from build123d import *

# Parameters (mm, degrees)
Y_KSEKLIK_EKSTR_ZYON1_DEPTH = 9
IZIM2_R                     = 1
KES_EKSTR_ZYON1_DEPTH       = 9
L_EK1_SCALE                 = 0.5


with BuildPart() as part:
    # Çizim1 → Yükseklik-Ekstrüzyon1 (new body)
    with BuildSketch(Plane(origin=(0, 0, 0), x_dir=(1, 0, 0), z_dir=(0, 1, 0))):
        with BuildLine():
            Line((3.94, 0), (3.94, -1.970806212))
            ThreePointArc((3.94, -1.970806212), (4.455977206, -3.302963323), (5.734671586, -3.94))
            Line((5.734671586, -3.94), (11.94, -3.94))
            Line((11.94, -3.94), (11.94, -1.970806212))
            Line((11.94, -1.970806212), (7.888485675, -1.970806212))
            ThreePointArc((7.888485675, -1.970806212), (6.494915238, -1.393570437), (5.917679463, 0))
            ThreePointArc((5.917679463, 0), (0, 5.917679463), (-5.917679463, 0))
            ThreePointArc((-5.917679463, 0), (-6.494915238, -1.393570437), (-7.888485675, -1.970806212))
            Line((-7.888485675, -1.970806212), (-11.94, -1.970806212))
            Line((-11.94, -1.970806212), (-11.94, -3.941612423))
            Line((-11.94, -3.941612423), (-5.752940471, -3.941612423))
            ThreePointArc((-5.752940471, -3.941612423), (-4.462169762, -3.309726511), (-3.94, -1.970806212))
            Line((-3.94, -1.970806212), (-3.94, 0))
            ThreePointArc((-3.94, 0), (0, 3.94), (3.94, 0))
        make_face()
    extrude(amount=Y_KSEKLIK_EKSTR_ZYON1_DEPTH)

    # Çizim2 → Kes-Ekstrüzyon1 (cut)
    with BuildSketch(Plane(origin=(0, 0, 1.970806212), x_dir=(-1, 0, 0), z_dir=(0, 0, -1))):
        with Locations((-9.914242837, 6.75)):
            Circle(IZIM2_R)
        with Locations((-9.914242837, 2.25)):
            Circle(IZIM2_R)
        with Locations((9.914242837, 2.25)):
            Circle(IZIM2_R)
        with Locations((9.914242837, 6.75)):
            Circle(IZIM2_R)
    extrude(amount=-KES_EKSTR_ZYON1_DEPTH, mode=Mode.SUBTRACT)


with BuildPart() as part_1:
    # Ölçek1: scaled about (-0.001148425, 4.5, -0.117296344)
    add(part.part.scale(L_EK1_SCALE).moved(Location((-0.000574213, 2.25, -0.058648172))))


solid = part_1.part
Read the model definition and answer for the solid it produces. Units are mm, in the model's axes. A direction names the side the tool comes from. Coordinates: 2 decimals unless noted, no trailing zeros. Order: outer loops, then holes, each group sorted by start corner. A loop starts at its lowest first (then second) coordinate and runs counter-clockwise, first axis right, second up. Notation, with made-up numbers: (77, 38.25) -> (117, 38.25) arc R22 cw to (117, 74.25) -> close; hole circle Ø4 at (77, 3.5). An arc over 180 degrees is marked (long way). Answer as a JSON object with one key per item and string values.
1) A cutting plane is placed at C-C, the plane y = 4.3. Determine the outline of the cut face in (x, z).
Model answer:
{"outline": "(-5.97, 0.93) -> (-3.94, 0.93) arc R0.99 cw to (-2.96, -0.06) arc R2.96 ccw to (2.96, -0.06) arc R0.99 cw to (3.94, 0.93) -> (5.97, 0.93) -> (5.97, 1.91) -> (2.87, 1.91) arc R0.99 ccw to (1.97, 0.93) -> (1.97, -0.06) arc R1.97 cw to (-1.97, -0.06) -> (-1.97, 0.93) arc R0.99 ccw to (-2.88, 1.91) -> (-5.97, 1.91) -> close"}
2) A cutting plane is placed at D-D, the plane z = -1.1. Determine the outline of the cut face in (x, y), plus the area to 3 significant figures.
Model answer:
{"outline": "(-2.77, 2.25) -> (-1.67, 2.25) -> (-1.67, 6.75) -> (-2.77, 6.75) -> close; (1.67, 2.25) -> (2.77, 2.25) -> (2.77, 6.75) -> (1.67, 6.75) -> close", "area": "9.88 mm²"}
3) The mould has two halves that part along Y. Classify faces 1 (the face through (4.48, 5.78, 1.41)), 2 (the face through (-2, 2.25, -1)), 3 (the face through (-2, 6.75, -1)), 4 (the face through (5, 4.5, 0.927)): released by +Y, released by -Y, zero draft, split by the parting line, or undercut.
Model answer:
{"face 1": "undercut", "face 2": "released by -Y", "face 3": "released by +Y", "face 4": "zero draft"}
4) A cutting plane is placed at A-A, the plane z = 1.15. Determine the outline of the cut face in (x, y) (3 decimals), plus the area to 3 significant figures.
Model answer:
{"outline": "(-5.971, 2.25) -> (-1.996, 2.25) -> (-1.996, 6.75) -> (-5.971, 6.75) -> close; (1.995, 2.25) -> (5.969, 2.25) -> (5.969, 6.75) -> (1.995, 6.75) -> close; hole circle Ø1 at (-4.958, 3.375); hole circle Ø1 at (-4.958, 5.625); hole circle Ø1 at (4.957, 3.375); hole circle Ø1 at (4.957, 5.625)", "area": "32.6 mm²"}
5) Each of these flat-tipped pins is pushed along its axis until it touches: pin 1 (0.5 mm diameter, centred on y = 4.5, z = 0, fed in from -X); pin 2 (2 mm diameter, centred on x = 5, y = 5, fed in from -Z); pin 3 (2 mm diameter, centred on x = -4.5, y = 3.5, fed in from -Z). Where does it stop, or does it pass through?
Model answer:
{"pin 1": "stops at x = -3.01", "pin 2": "stops at z = 0.93", "pin 3": "stops at z = 0.82"}
6) A tool of negligible diameter and unlimited length cuts with its end or side. For faces 5 (the face through (1.969, 4.5, 0.4)), 6 (the face through (0.064, 4.469, -3.017)), 7 (the face through (-4.9, 4.5, 0.927)), from which of +Z, -Z, +X, -X, +Y, -Y can it reach the whole face along a straight path? Write none if from no direction.
Model answer:
{"face 5": "+Z, +Y, -Y", "face 6": "-Z, +Y, -Y", "face 7": "-Z, -X, +Y, -Y"}
7) Consider line 1 along X through (y, z) = (3.8, -1.05); line 2 along Z through (x, y) = (4.75, 2.65); line 3 along X through (y, z) = (5.4, 1.2). Determine where each line is inside the solid, lowest interval first. Write a range as from..to.
Model answer:
{"line 1": "x = -2.79..-1.7, 1.7..2.79", "line 2": "z = 0.93..1.91", "line 3": "x = -5.97..-5.4, -4.51..-2.01, 2.01..4.51, 5.4..5.97"}
8) A cutting plane is placed at B-B, the plane y = 5.5. Determine the outline of the cut face in (x, z).
Model answer:
{"outline": "(-5.97, 0.93) -> (-5.44, 0.93) -> (-5.44, 1.91) -> (-5.97, 1.91) -> close; (-4.47, 0.93) -> (-3.94, 0.93) arc R0.99 cw to (-2.96, -0.06) arc R2.96 ccw to (2.96, -0.06) arc R0.99 cw to (3.94, 0.93) -> (4.47, 0.93) -> (4.47, 1.91) -> (2.87, 1.91) arc R0.99 ccw to (1.97, 0.93) -> (1.97, -0.06) arc R1.97 cw to (-1.97, -0.06) -> (-1.97, 0.93) arc R0.99 ccw to (-2.88, 1.91) -> (-4.47, 1.91) -> close; (5.44, 0.93) -> (5.97, 0.93) -> (5.97, 1.91) -> (5.44, 1.91) -> close"}
